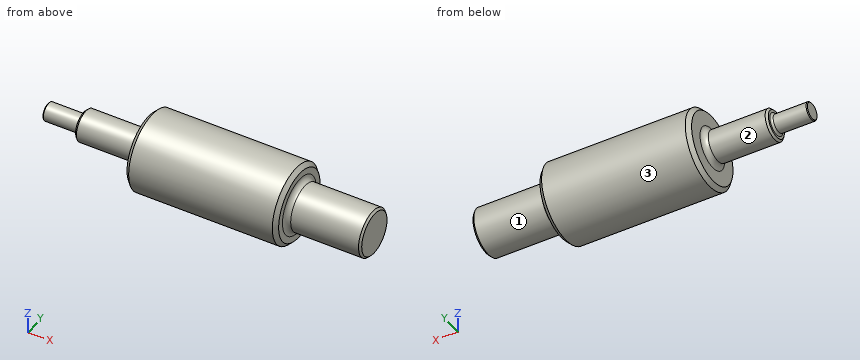
```python
from build123d import *

# Parameters (mm, degrees)
F2_SIZE = 2.54
F3_SIZE = 2.54
F4_SIZE = 1.27
F5_SIZE = 0.508
F6_SIZE = 1.27


with BuildPart() as f1:
    # F0 (on Front) → F1 (revolve)
    with BuildSketch(Plane.XZ):
        with BuildLine():
            Line((-58.015915, 9.94281), (-95.500656, 9.94281))
            Line((-95.500656, 9.94281), (-95.500656, 7.037411))
            ThreePointArc((-95.500656, 7.037411), (-95.887981, 6.102325), (-96.823067, 5.715))
            Line((-96.823067, 5.715), (-118.297269, 5.715))
            Line((-118.297269, 5.715), (-118.297269, 0))
            Line((-118.297269, 0), (89.53189, 0))
            Line((89.53189, 0), (89.53189, 14.916802))
            Line((89.53189, 14.916802), (45.083549, 14.916802))
            ThreePointArc((45.083549, 14.916802), (42.748683, 15.883936), (41.781549, 18.218802))
            Line((41.781549, 18.218802), (41.781549, 24.864788))
            Line((41.781549, 24.864788), (-54.713915, 24.864788))
            Line((-54.713915, 24.864788), (-54.713915, 13.24481))
            ThreePointArc((-54.713915, 13.24481), (-55.681049, 10.909944), (-58.015915, 9.94281))
        make_face()
    revolve(axis=Axis((-14.38269, 0, 0), (1, 0, 0)))

    # F2
    f2_edges = [f1.edges().sort_by_distance(p)[0] for p in [
        (41.781549, 0, -24.864788),
    ]]
    chamfer(f2_edges, length=F2_SIZE)

    # F3
    f3_edges = [f1.edges().sort_by_distance(p)[0] for p in [
        (-54.713915, 0, -24.864788),
    ]]
    chamfer(f3_edges, length=F3_SIZE)

    # F4
    f4_edges = [f1.edges().sort_by_distance(p)[0] for p in [
        (-95.500656, 0, -9.94281),
    ]]
    chamfer(f4_edges, length=F4_SIZE)

    # F5
    f5_edges = [f1.edges().sort_by_distance(p)[0] for p in [
        (-118.297269, 0, -5.715),
    ]]
    chamfer(f5_edges, length=F5_SIZE)

    # F6
    f6_edges = [f1.edges().sort_by_distance(p)[0] for p in [
        (89.53189, 0, -14.916802),
    ]]
    chamfer(f6_edges, length=F6_SIZE)


solid = f1.part
```
Can you work these out from the model? Positions are in its coordinate system, mm. Face numbers are marked on the shaded views. A direction names the side the tool comes from. Coordinates: 2 decimals unless noted, no trailing zeros. Loops run counter-clockwise (first coordinate to the right, second up) from the corner with the lowest first, then second, coordinate; pieces in that order, holes last.
1) Imagine slicing it at C-C on x = -2.5. List the corners of the cut face in (y, z) for me, plus the area to 3 significant figures.
2) Imagine slicing it at D-D on x = -60. List the corners of the cut face in (y, z) for me, plus the area to 3 significant figures.
3) For pin 1 (2 mm diameter, centred on x = 23, z = -17.5, fed in from +Y); pin 2 (12 mm diameter, centred on x = -44, y = -13.5, fed in from +Z); pin 3 (2 mm diameter, centred on y = 8.5, z = -11.5, fed in from -X), each with a flat end and sliding along its axis, tell me the tip position at first contact or that it passes through.
4) Which directions (+Z, -Z, +X, -X, +Y, -Y) give clear straight access to the entire face, cutting with the end or side of a thin tool? Please do the marked faces 1, 2 and 3.
5) I need wall thicknesses on probe 1 along X at (y, z) = (5.5, 5); probe 2 along Z at (x, y) = (-65.5, 7); probe 3 along Z at (x, y) = (20, -11). Which ranges of each line are inside material? Lowest first, please.
Completed:
1. outline: circle Ø49.73 at (0, 0)
1. area: 1,940 mm2
2. outline: circle Ø19.89 at (0, 0)
2. area: 311 mm2
3. pin 1: stops at y = 18.6
3. pin 2: stops at z = 23.71
3. pin 3: stops at x = -54.71
4. face 1: +X
4. face 2: -X
4. face 3: +X, -X
5. probe 1: x = -95.5 to 89.53
5. probe 2: z = -7.06 to 7.06
5. probe 3: z = -22.3 to 22.3
